from build123d import *

# Parameters (mm, degrees)
CROQUIS_PERILLA_R    = 12
CUERPO_DEPTH         = 9
MOLETEADO_DEPTH      = 20.209372712
MOLETEADO_DEPTH_BACK = 20.209372712
CROQUIS_MOLETEADO_R  = 2
CROQUIS_ARANDELA_R   = 5.5
ARANDELA_DEPTH       = 2
PASO_M4_DEPTH        = 20.001461932
PASO_M4_DEPTH_BACK   = 20.001461932
CROQUIS_PASO_R       = 2.2
CABEZA_M4_DEPTH      = 3.5


with BuildPart() as part:
    # Croquis_perilla → Cuerpo (new body)
    with BuildSketch(Plane(origin=(0, 0, 0), x_dir=(1, 0, 0), z_dir=(0, 1, 0))):
        with Locations(Location((0, 0, 0), (0, 0, 270))):
            Circle(CROQUIS_PERILLA_R)
    extrude(amount=CUERPO_DEPTH)

    # Croquis_moleteado → Moleteado (cut, two sides: drawn at the far end of the back side and taken through both)
    with BuildSketch(Plane(origin=(0, 0, 0), x_dir=(1, 0, 0), z_dir=(0, 1, 0)).offset(-MOLETEADO_DEPTH_BACK)):
        with Locations((12, 0)):
            Circle(CROQUIS_MOLETEADO_R)
        with Locations((10.392304845, 6)):
            Circle(CROQUIS_MOLETEADO_R)
        with Locations((6, 10.392304845)):
            Circle(CROQUIS_MOLETEADO_R)
        with Locations((0, 12)):
            Circle(CROQUIS_MOLETEADO_R)
        with Locations((-6, 10.392304845)):
            Circle(CROQUIS_MOLETEADO_R)
        with Locations((-10.392304845, 6)):
            Circle(CROQUIS_MOLETEADO_R)
        with Locations((-12, 0)):
            Circle(CROQUIS_MOLETEADO_R)
        with Locations((-10.392304845, -6)):
            Circle(CROQUIS_MOLETEADO_R)
        with Locations((-6, -10.392304845)):
            Circle(CROQUIS_MOLETEADO_R)
        with Locations((0, -12)):
            Circle(CROQUIS_MOLETEADO_R)
        with Locations((6, -10.392304845)):
            Circle(CROQUIS_MOLETEADO_R)
        with Locations((10.392304845, -6)):
            Circle(CROQUIS_MOLETEADO_R)
    extrude(amount=MOLETEADO_DEPTH + MOLETEADO_DEPTH_BACK, mode=Mode.SUBTRACT)

    # Croquis_arandela → Arandela (add)
    with BuildSketch(Plane(origin=(0, 0, 0), x_dir=(1, 0, 0), z_dir=(0, 1, 0))):
        with Locations(Location((0, 0, 0), (0, 0, 270))):
            Circle(CROQUIS_ARANDELA_R)
    extrude(amount=-ARANDELA_DEPTH)

    # Croquis_paso → Paso_M4 (cut, two sides: drawn at the far end of the back side and taken through both)
    with BuildSketch(Plane(origin=(0, 0, 0), x_dir=(1, 0, 0), z_dir=(0, 1, 0)).offset(-PASO_M4_DEPTH_BACK)):
        with Locations(Location((0, 0, 0), (0, 0, 270))):
            Circle(CROQUIS_PASO_R)
    extrude(amount=PASO_M4_DEPTH + PASO_M4_DEPTH_BACK, mode=Mode.SUBTRACT)

    # Croquis_cabeza → Cabeza_M4 (cut)
    with BuildSketch(Plane(origin=(0, 9, 0), x_dir=(1, 0, 0), z_dir=(0, 1, 0))):
        Polygon((4.156921938, 0), (2.078460969, 3.6), (-2.078460969, 3.6), (-4.156921938, 0), (-2.078460969, -3.6), (2.078460969, -3.6), align=None)
    extrude(amount=-CABEZA_M4_DEPTH, mode=Mode.SUBTRACT)


solid = part.part
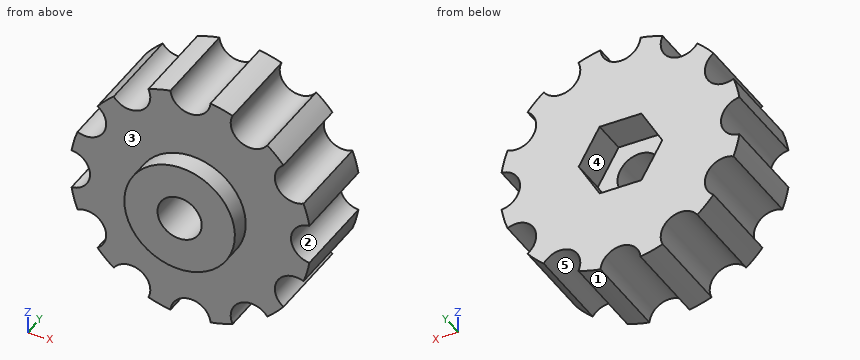
The model under review builds one solid part; all positions refer to its coordinate system, in mm. Face numbers are marked on the shaded views. A direction names the side the tool comes from. Round coordinates to 2 decimals unless told otherwise and drop trailing zeros. Order: outer loops, then holes, each group sorted by start corner. A loop starts at its lowest first (then second) coordinate and runs counter-clockwise, first axis right, second up. Notation, with made-up numbers: (24, -32.75) -> (73, -32.75) arc R20 cw to (73, -11.75) -> close; hole circle Ø3 at (-12.75, 29). An arc over 180 degrees is marked (long way). Use CSV: the item, a comma, the result in double quotes. Start each with the question number.
(1) Tool access review of the marked faces 4 and 5: name each direction out of +Z, -Z, +X, -X, +Y, -Y from which nothing blocks a thin tool from reaching the whole face with its end or side.
(2) Consider section B-B on y = 1.25. Write out the cut boundary in (x, z).
(3) Mouldability with a two-part tool opening along Z and no side actions: class the marked faces 1, 2 and 3 as pulls with the +Z half, pulls with the -Z half, needs draft (parallel to the pull), parting line crosses it, or undercut.
(4) Wall thickness on probe 1 along X at (y, z) = (4.25, 0); probe 2 along Y at (x, z) = (-8.75, -7.25); probe 3 along Z at (x, y) = (-0.25, 6.25): over which ranges is each line inside the solid? List them lowest first. Write a range as from..to.
(5) Insertion check: pin 1 (5 mm diameter, centred on x = 9.5, y = 5.5, fed in from +Z); pin 2 (3.5 mm diameter, centred on x = -0.5, z = -1.5, fed in from +Y); pin 3 (3 mm diameter, centred on x = -7.5, y = 0, fed in from +Z). Each pin has a flat end and moves straight along its axis. Give the tip position at first contact, or say it passes through.
(6) Consider section A-A on x = 0. Write out the cut boundary in (y, z).
Responses:
1,face 4,"+Y"
1,face 5,"+Y, -Y"
2,outline,"(-11.83, -1.99) arc R12 ccw to (-11.24, -4.19) arc R2 cw to (-9.25, -7.64) arc R12 ccw to (-7.64, -9.25) arc R2 cw to (-4.19, -11.24) arc R12 ccw to (-1.99, -11.83) arc R2 cw to (1.99, -11.83) arc R12 ccw to (4.19, -11.24) arc R2 cw to (7.64, -9.25) arc R12 ccw to (9.25, -7.64) arc R2 cw to (11.24, -4.19) arc R12 ccw to (11.83, -1.99) arc R2 cw to (11.83, 1.99) arc R12 ccw to (11.24, 4.19) arc R2 cw to (9.25, 7.64) arc R12 ccw to (7.64, 9.25) arc R2 cw to (4.19, 11.24) arc R12 ccw to (1.99, 11.83) arc R2 cw to (-1.99, 11.83) arc R12 ccw to (-4.19, 11.24) arc R2 cw to (-7.64, 9.25) arc R12 ccw to (-9.25, 7.64) arc R2 cw to (-11.24, 4.19) arc R12 ccw to (-11.83, 1.99) arc R2 cw to start; hole circle Ø4.4 at (0, 0)"
3,face 1,"pulls with the -Z half"
3,face 2,"undercut"
3,face 3,"needs draft"
4,probe 1,"-10..-2.2, 2.2..10"
4,probe 2,"0..9"
4,probe 3,"-10.02..-3.6, 3.6..10.02"
5,pin 1,"z = 9.25"
5,pin 2,"y = 5.5"
5,pin 3,"z = 9.25"
6,outline,"(-2, -5.5) -> (0, -5.5) -> (0, -10) -> (9, -10) -> (9, -3.6) -> (5.5, -3.6) -> (5.5, -2.2) -> (-2, -2.2) -> close; (-2, 2.2) -> (5.5, 2.2) -> (5.5, 3.6) -> (9, 3.6) -> (9, 10) -> (0, 10) -> (0, 5.5) -> (-2, 5.5) -> close"
